Read the model definition and answer for the solid it produces. Units are mm, in the model's axes. A direction names the side the tool comes from. Give positions to 0.01 mm unless a question says otherwise; leave off trailing zeros. Loops run counter-clockwise (first coordinate to the right, second up) from the corner with the lowest first, then second, coordinate; pieces in that order, holes last. Notation, with made-up numbers: (40, -9) - (89, -9) arc R29 cw to (89, 22) - close; hole circle Ø6 at (79, 63.25). An arc over 180 degrees is marked (long way). Use a Markdown table: item, result. Add a question column.
Item 1: For a pull along Y with two mould halves and no side action, classify faces 6 (the face through (-11.99, 4.57, 5.01)), 7 (the face through (-11, 2.749, 2)), 8 (the face through (-11.125, 6.401, 5.263)) as +Y half, -Y half, draft (parallel to the pull), parting line (faces both ways), or undercut.
Item 2: A cutting plane is placed at B-B (x = -0.75). Determine the outline of the cut face in (y, z).
Item 3: A cutting plane is placed at A-A (y = -13.25). Determine the outline of the cut face in (x, z).
Item 4: A cutting plane is placed at C-C (y = 3.5). Determine the outline of the cut face in (x, z).
Item 5: Which of the six approach directions +Z, -Z, +X, -X, +Y, -Y give full straight-line access (tool end or side, diameter ignored) to faces 1 (the face through (-12.075, 1.481, 6.408)), 2 (the face through (-8.302, 1, 4)), 3 (the face through (6.84, 4.57, 4.9)), 4 (the face through (6.93, 1.48, 6.42)), 5 (the face through (-3.54, 5.05, 5.64))?
Item 6: Each of these flat-tipped pins is pushed along its axis until it touches: P1, Ø2.5, axis at y = -11.5, z = 5.5, coming from the +X side; P2, Ø5, axis at x = 1.5, z = 3, coming from the +Y side; P3, Ø0.8, axis at y = 1.5, z = 4, coming from the +X side. Where does it stop, or does it pass through?
Item 7: Consider probe 1 along Y at (x, z) = (6.2, 6.5); probe 2 along Y at (x, z) = (6.9, 6.5); probe 3 along X at (y, z) = (0.5, 3). Determine where each line is inside the solid, lowest interval first. Write a range as [from, to].
from build123d import *

# Parameters (mm, degrees)
ESQUISSE1_W               = 21.5
ESQUISSE1_H               = 15
EXTRUSION1_DEPTH          = 10
EXTRUSION2_DEPTH          = 2.5
ESQUISSE4_R               = 1.75
EXTRUSION3_DEPTH          = 3.9
ESQUISSE7_R               = 0.25
EXTRUSION4_DEPTH          = 5
ESQUISSE8_R               = 4.580355977
ESQUISSE8_R_2             = 4.37854461
ENL_V_MAT_EXTRU_3_DEPTH   = 0.2
TROU_TARAUD_M3X0_52_D     = 2.5
TROU_TARAUD_M3X0_52_DEPTH = 5.5
TROU_TARAUD_M3X0_52_TIP   = 0.751075774


with BuildPart() as part:
    # Esquisse1 → Extrusion1 (new body)
    with BuildSketch(Plane.XY):
        with Locations((-2.605785234, -7.251083667)):
            Rectangle(ESQUISSE1_W, ESQUISSE1_H)
    extrude(amount=EXTRUSION1_DEPTH)

    # Esquisse2 → Extrusion2 (add)
    with BuildSketch(Plane(origin=(0, 0.248916333, 0), x_dir=(-1, 0, 0), z_dir=(0, 1, 0))):
        Polygon((13.309313152, 5.695412518), (10.805785234, 7.140825036), (8.302257315, 5.695412518), (8.302257315, 2.804587482), (10.805785234, 1.359174964), (13.309313152, 2.804587482), align=None)
        Polygon((6.076207844, 6.801050244), (3.131722221, 6.798948457), (1.661299611, 4.247898212), (3.135362624, 1.698949756), (6.079848247, 1.701051543), (7.550270856, 4.252101788), align=None)
        Polygon((-3.097880639, 5.811510782), (-5.698355708, 7.192644162), (-8.194689836, 5.63113338), (-8.090548894, 2.688489218), (-5.490073824, 1.307355838), (-2.993739697, 2.86886662), align=None)
    extrude(amount=EXTRUSION2_DEPTH)

    # Esquisse4 → Extrusion3 (add)
    with BuildSketch(Plane(origin=(0, 2.748916333, 0), x_dir=(-1, 0, 0), z_dir=(0, 1, 0))):
        with Locations(Location((10.805785234, 4.25, 0), (0, 0, 90))):
            Circle(ESQUISSE4_R)
        with Locations(Location((4.605785234, 4.25, 0), (0, 0, 270))):
            Circle(ESQUISSE4_R)
        with Locations(Location((-5.594214766, 4.25, 0), (0, 0, 270))):
            Circle(ESQUISSE4_R)
    extrude(amount=EXTRUSION3_DEPTH)

    # Esquisse7 → Extrusion4 (add)
    with BuildSketch(Plane(origin=(8.144214766, 0, 0), x_dir=(0, 0, -1), z_dir=(1, 0, 0))):
        with Locations(Location((-3.56, -11.101083667, 0), (0, 0, 270))):
            Circle(ESQUISSE7_R)
        with Locations(Location((-7, -11.101083667, 0), (0, 0, 270))):
            Circle(ESQUISSE7_R)
    extrude(amount=EXTRUSION4_DEPTH)

    # Esquisse8 → Enl_v. mat.-Extru.3 (cut)
    with BuildSketch(Plane(origin=(8.144214766, 0, 0), x_dir=(0, 0, -1), z_dir=(1, 0, 0))):
        with Locations(Location((-5, -9.777233514, 0), (0, 0, 90))):
            Circle(ESQUISSE8_R)
        with Locations(Location((-5, -9.777233514, 0), (0, 0, 90))):
            Circle(ESQUISSE8_R_2, mode=Mode.SUBTRACT)
    extrude(amount=-ENL_V_MAT_EXTRU_3_DEPTH, mode=Mode.SUBTRACT)

    # Trou taraud_ M3x0.52
    with Locations(Plane(origin=(8.144214766, -3.751083667, 6.5), x_dir=(0, 1, 0), z_dir=(1, 0, 0))):
        with Locations((0, 0)):
            Hole(TROU_TARAUD_M3X0_52_D / 2, depth=TROU_TARAUD_M3X0_52_DEPTH)
            with Locations((0, 0, -(TROU_TARAUD_M3X0_52_DEPTH + TROU_TARAUD_M3X0_52_TIP / 2))):  # 118° drill point
                Cone(0, TROU_TARAUD_M3X0_52_D / 2, TROU_TARAUD_M3X0_52_TIP, mode=Mode.SUBTRACT)

    # Esquisse13 → Enl_vement de mati_re-R_volution1 (revolve, cut)
    with BuildSketch(Plane.XY.offset(4.25), mode=Mode.PRIVATE) as enl_vement_de_mati_re_r_volution1_sk:
        Polygon((-9.744077061, 6.648916333), (-9.744077061, 6.159304946), (-9.055785234, 5.295659421), (-9.055785234, 4.809098562), (-9.399931147, 4.809098562), (-9.399931147, 4.334701724), (-9.055785234, 4.091421295), (-9.055785234, 2.748916333), (-8.612823064, 2.748916333), (-8.612823064, 6.648916333), align=None)
    revolve(enl_vement_de_mati_re_r_volution1_sk.sketch.rotate(Axis((-10.805785234, 6.648916333, 4.25), (0, -1, 0)), 90), axis=Axis((-10.805785234, 6.648916333, 4.25), (0, -1, 0)), mode=Mode.SUBTRACT)

    # Esquisse14 → Enl_vement de mati_re-R_volution2 (revolve, cut)
    with BuildSketch(Plane.XY.offset(4.25), mode=Mode.PRIVATE) as enl_vement_de_mati_re_r_volution2_sk:
        Polygon((-3.544077061, 6.648916333), (-3.544077061, 6.159304946), (-2.855785234, 5.295659421), (-2.855785234, 4.809098562), (-3.199931147, 4.809098562), (-3.199931147, 4.334701724), (-2.855785234, 4.091421295), (-2.855785234, 2.748916333), (-2.412823064, 2.748916333), (-2.412823064, 6.648916333), align=None)
    revolve(enl_vement_de_mati_re_r_volution2_sk.sketch.rotate(Axis((-4.605785234, 6.648916333, 4.25), (0, -1, 0)), 90), axis=Axis((-4.605785234, 6.648916333, 4.25), (0, -1, 0)), mode=Mode.SUBTRACT)

    # Esquisse15 → Enl_vement de mati_re-R_volution3 (revolve, cut)
    with BuildSketch(Plane.XY.offset(4.25), mode=Mode.PRIVATE) as enl_vement_de_mati_re_r_volution3_sk:
        Polygon((6.655922939, 6.648916333), (6.655922939, 6.159304946), (7.344214766, 5.295659421), (7.344214766, 4.809098562), (7.000068853, 4.809098562), (7.000068853, 4.334701724), (7.344214766, 4.091421295), (7.344214766, 2.748916333), (7.787176936, 2.748916333), (7.787176936, 6.648916333), align=None)
    revolve(enl_vement_de_mati_re_r_volution3_sk.sketch.rotate(Axis((5.594214766, 6.648916333, 4.25), (0, -1, 0)), 90), axis=Axis((5.594214766, 6.648916333, 4.25), (0, -1, 0)), mode=Mode.SUBTRACT)


solid = part.part
Geometry says:
| question | item | result |
|---|---|---|
| 1 | face 6 | undercut |
| 1 | face 7 | +Y half |
| 1 | face 8 | draft |
| 2 | outline | (-14.75, 0) - (0.25, 0) - (0.25, 10) - (-14.75, 10) - close |
| 3 | outline | (-13.36, 0) - (8.14, 0) - (8.14, 2.01) - (7.94, 2.01) - (7.94, 2.33) - (8.14, 2.33) - (8.14, 7.67) - (7.94, 7.67) - (7.94, 7.99) - (8.14, 7.99) - (8.14, 10) - (-13.36, 10) - close |
| 4 | outline | circle Ø3.5 at (-10.81, 4.25); circle Ø3.5 at (-4.61, 4.25); circle Ø3.5 at (5.59, 4.25) |
| 5 | face 1 | +Z, -X, +Y |
| 5 | face 2 | +Z, -Z, +Y |
| 5 | face 3 | none |
| 5 | face 4 | +Z, +X, +Y |
| 5 | face 5 | +Y |
| 6 | P1 | x = 8.14 |
| 6 | P2 | y = 2.75 |
| 6 | P3 | x = 8.15 |
| 7 | probe 1 | [-14.75, -5], [-2.5, 2.75] |
| 7 | probe 2 | [-14.75, -5], [-2.5, 0.25] |
| 7 | probe 3 | [-13.31, -8.3], [-6.83, -2.38], [3, 8.1] |
